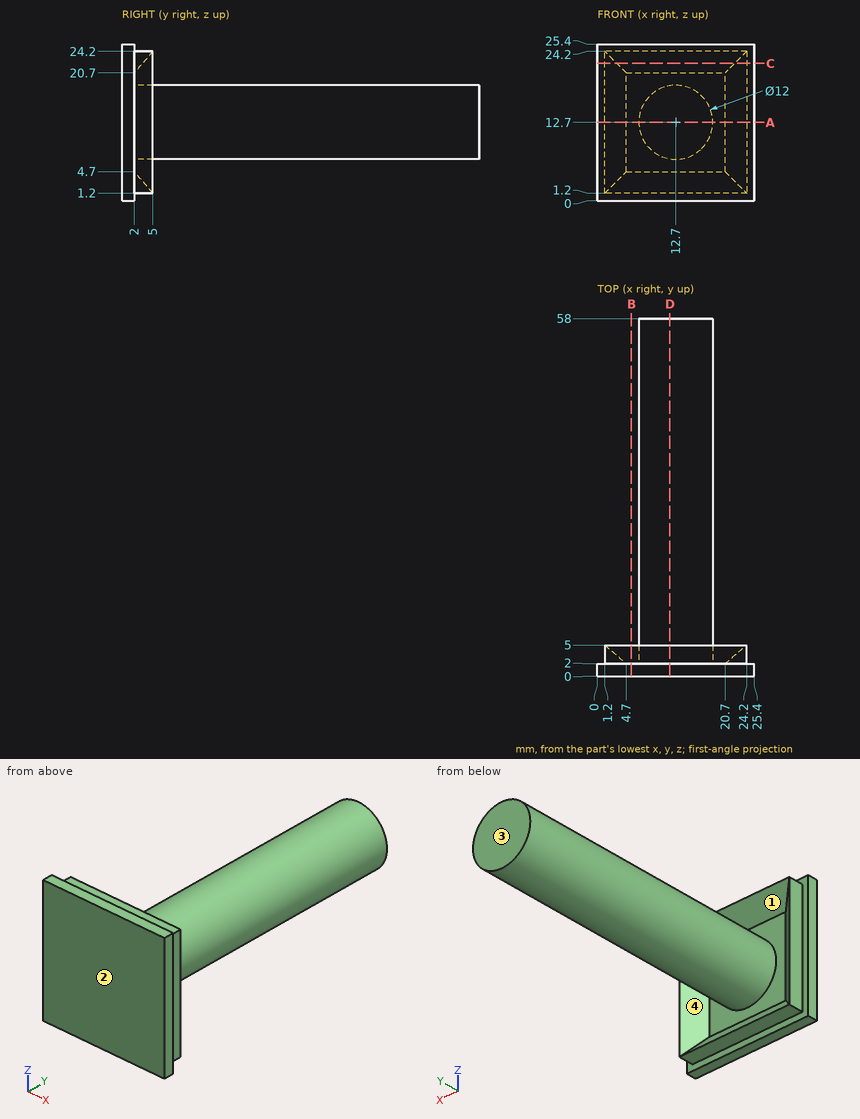
Study the drawing (mm; zero at the part's minimum x, y, z) and answer. A direction names the side the tool comes from. Coordinates: 2 decimals unless noted, no trailing zeros. Write each loop counter-clockwise with the first axis right and the second up, starting at its lowest first coordinate (ties: lowest second). Pieces come first, ordered by that corner, then holes. Notation, with made-up numbers: (84.25, -27) - (142.25, -27) arc R10 ccw to (142.25, -18) - close; hole circle Ø1 at (33.5, 56). An arc over 180 degrees is marked (long way). Return JSON: item names as keys, results as strings. Group by question number.
1. Which of the six approach directions +Z, -Z, +X, -X, +Y, -Y give full straight-line access (tool end or side, diameter ignored) to the marked faces 3 and 4?
2. A cutting plane is placed at A-A, the plane z = 12.7. Determine the outline of the cut face in (x, y), plus the area to 3 significant figures.
3. A cutting plane is placed at C-C, the plane z = 22.25. Determine the outline of the cut face in (x, y), plus the area to 3 significant figures.
4. A cutting plane is placed at D-D, the plane x = 11.75. Determine the outline of the cut face in (y, z), plus the area to 3 significant figures.
5. Determine the mould class of the marked faces 1 and 2 for opening direction Z: released by +Z, released by -Z, zero draft, split by the parting line, or undercut.
6. Straight lines are drawn through the part: L1, parallel to Z at x = 13, y = 9.5; L2, parallel to Y at x = 24.25, z = 11; L3, parallel to X at y = 4, z = 5.75. For each, find the intervals that lie inside material, in ascending order.
7. A cutting plane is placed at B-B, the plane x = 5.5. Determine the outline of the cut face in (y, z).
8. Given pin 1 (1.5 mm diameter, centred on y = 9, z = 17.5, fed in from +X); pin 2 (2.5 mm diameter, centred on y = 3.5, z = 12.5, fed in from +X); pin 3 (1.5 mm diameter, centred on y = 49, z = 10.5, fed in from +X), each flat-ended and moving along its own axis, determine where each tip first touches the part or whether it passes through.
Ans:
{
 "1": {"face 3": "+Z, -Z, +X, -X, +Y", "face 4": "+Y"},
 "2": {"outline": "(0, 0) - (25.4, 0) - (25.4, 2) - (24.2, 2) - (24.2, 5) - (20.7, 2) - (18.7, 2) - (18.7, 58) - (6.7, 58) - (6.7, 2) - (4.7, 2) - (1.2, 5) - (1.2, 2) - (0, 2) - close", "area": "733 mm²"},
 "3": {"outline": "(0, 0) - (25.4, 0) - (25.4, 2) - (24.2, 2) - (24.2, 5) - (22.25, 3.33) - (3.15, 3.33) - (1.2, 5) - (1.2, 2) - (0, 2) - close", "area": "84.6 mm²"},
 "4": {"outline": "(0, 0) - (2, 0) - (2, 1.2) - (5, 1.2) - (2, 4.7) - (2, 6.78) - (58, 6.78) - (58, 18.62) - (2, 18.62) - (2, 20.7) - (5, 24.2) - (2, 24.2) - (2, 25.4) - (0, 25.4) - close", "area": "725 mm²"},
 "5": {"face 1": "undercut", "face 2": "zero draft"},
 "6": {"L1": "6.71 to 18.69", "L2": "0 to 2", "L3": "1.2 to 2.37, 23.03 to 24.2"},
 "7": {"outline": "(0, 0) - (2, 0) - (2, 1.2) - (5, 1.2) - (2, 4.7) - (2, 20.7) - (5, 24.2) - (2, 24.2) - (2, 25.4) - (0, 25.4) - close"},
 "8": {"pin 1": "x = 17.13", "pin 2": "x = 24.2", "pin 3": "x = 18.52"}
}
